Input: part model. Units: mm. Frame: model coordinates. Round coordinates to 2 decimals unless told otherwise and drop trailing zeros. Loops run counter-clockwise (first coordinate to the right, second up) from the corner with the lowest first, then second, coordinate; pieces in that order, holes last.
1) Ray query, line 1 along Z through (x, y) = (-7.25, 10); line 2 along Z through (x, y) = (-7.35, 10); line 3 along Y through (x, z) = (-3, 128.5). Return the intervals inside material, ascending.
2) Draft query along Y for faces 1 (the face through (-6, 7, 148)), 2 (the face through (-6.2, 10.1, 0)), 3 (the face through (-4, 0, 148)). Return one class per face: pulls with the +Y half, pulls with the -Y half, needs draft (parallel to the pull), parting line crosses it, or undercut.
3) First-contact query: pin 1 (4 mm diameter, centred on y = 10, z = 150, fed in from +X); pin 2 (1.5 mm diameter, centred on x = -4, y = 7, fed in from -Z). Flat tips, straight axial feed; report the tip coordinate or a pass-through.
4) Section A-A, the plane x = -2. Return loops of the section in (y, z).
5) Section B-B, the plane z = 173.5. Return loops of the section in (x, y) (3 decimals).
Autodesk Inventor part; units mm, degrees
ref_plane "to_rail_XY" through (0.6, 10, 150) normal (0, 0, 1) x (1, 0, 0)
ref_plane "to_rail_YZ" through (0.6, 10, 150) normal (1, 0, 0) x (0, 1, 0)
ref_plane "to_rail_ZX" through (0.6, 10, 150) normal (0, 1, 0) x (0, 0, 1)
sketch "Sketch_1" plane through (0, 0, 0) normal (0, 0, 1) x (1, 0, 0)
  line L0 (-7.4, 19.7) -> (-7.4, 0.3)
  arc A0 (-7.4, 0.3) -> (-7.1, 0) centre (-7.1, 0.3) ccw
  line L1 (-7.1, 0) -> (-0.3, 0)
  arc A1 (-0.3, 0) -> (0, 0.3) centre (-0.3, 0.3) ccw
  line L2 (0, 0.3) -> (0, 2.95)
  arc A2 (0, 2.95) -> (-0.2, 3.15) centre (-0.2, 2.95) ccw
  line L3 (-0.2, 3.15) -> (-0.5141, 3.15)
  arc A3 (-0.5141, 3.15) -> (-0.708, 2.999) centre (-0.5141, 2.95) ccw
  arc A4 (-4.392, 2.999) -> (-0.708, 2.999) centre (-2.55, 3.465) ccw
  arc A5 (-4.392, 2.999) -> (-4.5859, 3.15) centre (-4.5859, 2.95) ccw
  line L4 (-4.5859, 3.15) -> (-5.8, 3.15)
  arc A6 (-6, 3.35) -> (-5.8, 3.15) centre (-5.8, 3.35) ccw
  line L5 (-6, 3.35) -> (-6, 16.65)
  arc A7 (-5.8, 16.85) -> (-6, 16.65) centre (-5.8, 16.65) ccw
  line L6 (-5.8, 16.85) -> (-4.5859, 16.85)
  arc A8 (-4.5859, 16.85) -> (-4.392, 17.001) centre (-4.5859, 17.05) ccw
  arc A9 (-0.708, 17.001) -> (-4.392, 17.001) centre (-2.55, 16.535) ccw
  arc A10 (-0.708, 17.001) -> (-0.5141, 16.85) centre (-0.5141, 17.05) ccw
  line L7 (-0.5141, 16.85) -> (-0.2, 16.85)
  arc A11 (-0.2, 16.85) -> (0, 17.05) centre (-0.2, 17.05) ccw
  line L8 (0, 17.05) -> (0, 19.7)
  arc A12 (0, 19.7) -> (-0.3, 20) centre (-0.3, 19.7) ccw
  line L9 (-0.3, 20) -> (-7.1, 20)
  arc A13 (-7.1, 20) -> (-7.4, 19.7) centre (-7.1, 19.7) ccw
extrude "Extrusion1" add sketch "Sketch_1" along normal blind 300
sketch "Sketch2" plane through (-6, 3.35, 0) normal (1, 0, 0) x (0, 0, -1)
  point P0 (-15, 6.65)
hole "Hole1" at (-6, 10, 15) direction (-1, 0, 0) diameter 3.5 depth 1.4 countersink diameter 6.1 countersink angle 90
pattern_linear "Rectangular Pattern1" count 3 spacing 135 along (0, 0, 1) of "Hole1"
ref_plane "to_rail_XY" through (0.6, 10, 150) normal (0, 0, 1) x (1, 0, 0)
ref_plane "to_rail_YZ" through (0.6, 10, 150) normal (1, 0, 0) x (0, 1, 0)
ref_plane "to_rail_ZX" through (0.6, 10, 150) normal (0, 1, 0) x (0, 0, 1)
properties part number "SAR330-30_b"
Final values:
1. line 1: z = 0 to 13.2, 16.8 to 148.2, 151.8 to 283.2, 286.8 to 300
1. line 2: z = 0 to 13.25, 16.75 to 148.25, 151.75 to 283.25, 286.75 to 300
1. line 3: y = 0 to 1.62, 18.38 to 20
2. face 1: undercut
2. face 2: needs draft
2. face 3: pulls with the -Y half
3. pin 1: stops at x = -7.05
3. pin 2: passes through
4. outline: (0, 0) - (1.65, 0) - (1.65, 300) - (0, 300) - close; (18.35, 0) - (20, 0) - (20, 300) - (18.35, 300) - close
5. outline: (-7.4, 0.3) arc R0.3 ccw to (-7.1, 0) - (-0.3, 0) arc R0.3 ccw to (0, 0.3) - (0, 2.95) arc R0.2 ccw to (-0.2, 3.15) - (-0.514, 3.15) arc R0.2 ccw to (-0.708, 2.999) arc R1.9 cw to (-4.392, 2.999) arc R0.2 ccw to (-4.586, 3.15) - (-5.8, 3.15) arc R0.2 cw to (-6, 3.35) - (-6, 16.65) arc R0.2 cw to (-5.8, 16.85) - (-4.586, 16.85) arc R0.2 ccw to (-4.392, 17.001) arc R1.9 cw to (-0.708, 17.001) arc R0.2 ccw to (-0.514, 16.85) - (-0.2, 16.85) arc R0.2 ccw to (0, 17.05) - (0, 19.7) arc R0.3 ccw to (-0.3, 20) - (-7.1, 20) arc R0.3 ccw to (-7.4, 19.7) - close
